For this review, take the finished solid that the model builds, in its own axes (mm). Face numbers are marked on the shaded views. A direction names the side the tool comes from. Round coordinates to 2 decimals unless told otherwise and drop trailing zeros. Write each loop counter-clockwise with the first axis right and the second up, starting at its lowest first coordinate (ties: lowest second). Pieces come first, ordered by that corner, then holes. Notation, with made-up numbers: M 55.25,56.25 L 92.25,56.25 A20 ccw 92.25,91.25 Z; hole C -10,28 d1. An arc over 180 degrees is marked long. Answer in a Markdown table with one row per item.
```python
from build123d import *

# Parameters (mm, degrees)
BOSS_EXTRUDE7_DEPTH      = 12
BOSS_EXTRUDE7_DEPTH_BACK = 12
FILLET1_R                = 10
SKETCH1_R                = 3.98
BOSS_EXTRUDE3_DEPTH      = 10
SKETCH5_R                = 1.6
CUT_EXTRUDE1_DEPTH       = 165.414111317
SKETCH6_R                = 2
CUT_EXTRUDE2_DEPTH       = 3
SKETCH7_R                = 3.98
BOSS_EXTRUDE5_DEPTH      = 10
SKETCH9_R                = 1.6
CUT_EXTRUDE3_DEPTH       = 17
SKETCH10_R               = 4
CUT_EXTRUDE4_DEPTH       = 3


with BuildPart() as part:
    # Sketch11 → Boss-Extrude7 (new, two sides: drawn at the far end of the back side and taken through both)
    with BuildSketch(Plane.XY.offset(-BOSS_EXTRUDE7_DEPTH_BACK)):
        Polygon((-86.2, 142), (-86.2, 26), (-50.2, -10), (15.8, -10), (15.8, 0), (-46.057864376, 0), (-76.2, 30.142135624), (-76.2, 142), align=None)
    extrude(amount=BOSS_EXTRUDE7_DEPTH + BOSS_EXTRUDE7_DEPTH_BACK)

    # Fillet1
    fillet1_edges = [part.edges().sort_by_distance(p)[0] for p in [
        (-81.2, 142, -12),
        (15.8, -5, -12),
        (15.8, -5, 12),
        (-81.2, 142, 12),
    ]]
    fillet(fillet1_edges, radius=FILLET1_R)

    # Sketch1 → Boss-Extrude3 (add)
    with BuildSketch(Plane(origin=(-76.2, 0, 0), x_dir=(0, 0, -1), z_dir=(1, 0, 0))):
        with Locations((0, 128)):
            Circle(SKETCH1_R)
    extrude(amount=BOSS_EXTRUDE3_DEPTH)

    # Sketch5 → Cut-Extrude1 (cut, through all)
    with BuildSketch(Plane(origin=(-66.2, 0, 0), x_dir=(0, 0, -1), z_dir=(1, 0, 0))):
        with Locations((0, 128)):
            Circle(SKETCH5_R)
    extrude(amount=-CUT_EXTRUDE1_DEPTH, mode=Mode.SUBTRACT)

    # Sketch6 → Cut-Extrude2 (cut)
    with BuildSketch(Plane.ZY.offset(86.2)):
        with Locations((0, 128)):
            Circle(SKETCH6_R)
    extrude(amount=-CUT_EXTRUDE2_DEPTH, mode=Mode.SUBTRACT)

    # Sketch7 → Boss-Extrude5 (add)
    with BuildSketch(Plane(origin=(0, 0, 0), x_dir=(1, 0, 0), z_dir=(0, 1, 0))):
        with Locations(Location((-0.08822806, 0, 0), (0, 0, 270))):
            Circle(SKETCH7_R)
    extrude(amount=BOSS_EXTRUDE5_DEPTH)

    # Sketch9 → Cut-Extrude3 (cut)
    with BuildSketch(Plane(origin=(0, 10, 0), x_dir=(1, 0, 0), z_dir=(0, 1, 0))):
        with Locations(Location((-0.08822806, 0, 0), (0, 0, 270))):
            Circle(SKETCH9_R)
    extrude(amount=-CUT_EXTRUDE3_DEPTH, mode=Mode.SUBTRACT)

    # Sketch10 → Cut-Extrude4 (cut)
    with BuildSketch(Plane.XZ.offset(10)):
        with Locations(Location((-0.08822806, 0, 0), (0, 0, 270))):
            Circle(SKETCH10_R)
    extrude(amount=-CUT_EXTRUDE4_DEPTH, mode=Mode.SUBTRACT)


solid = part.part
```
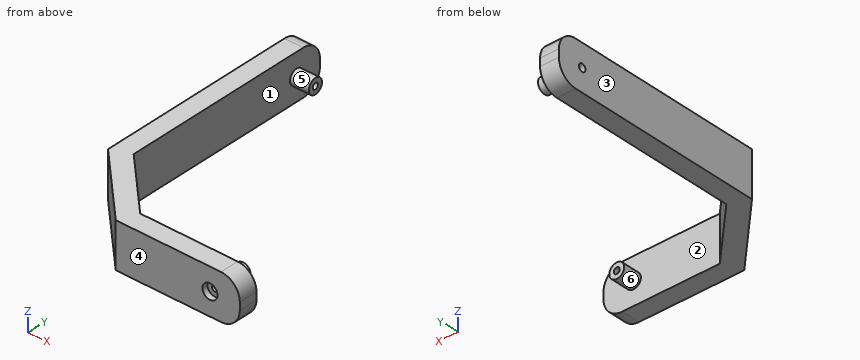
Q1. Take a section at C-C (z = 8.5). State the section outline as (x, y) points.
Found:
| item | result |
|---|---|
| outline | M -86.2,26 L -50.2,-10 L 13.4,-10 L 13.4,0 L -46.06,0 L -76.2,30.14 L -76.2,139.6 L -86.2,139.6 Z |
Q2. Take a section at A-A (y = 128). State the section outline as (x, z) points, then the cut area to 3 significant figures.
Found:
| item | result |
|---|---|
| outline | M -86.2,-12 L -76.2,-12 L -76.2,-3.98 L -66.2,-3.98 L -66.2,-1.6 L -83.2,-1.6 L -83.2,-2 L -86.2,-2 Z; M -86.2,2 L -83.2,2 L -83.2,1.6 L -66.2,1.6 L -66.2,3.98 L -76.2,3.98 L -76.2,12 L -86.2,12 Z |
| area | 253 mm² |
Q3. Take a section at B-B (z = 0). State how many separate pieces and enclosed holes the cut face has, then the cut area to 3 significant figures.
Found:
| item | result |
|---|---|
| separate pieces | 3 |
| enclosed holes | 0 |
| area | 2,260 mm² |
Q4. Mouldability with a two-part tool opening along Y and no side actions: class the marked faces 1, 2 and 3 as +Y half, -Y half, draft (parallel to the pull), parting line (faces both ways), or undercut.
Found:
| item | result |
|---|---|
| face 1 | undercut |
| face 2 | +Y half |
| face 3 | draft |
Q5. Take a section at D-D (y = 103). State the section outline as (x, z) points.
Found:
| item | result |
|---|---|
| outline | M -86.2,-12 L -76.2,-12 L -76.2,12 L -86.2,12 Z |
Q6. For probe 1 along X at (y, z) = (67.5, -10.5); probe 2 along Y at (x, z) = (-9, 2.75); probe 3 along Y at (x, z) = (1.5, -3.5), list the stretches that pass through material, from the lowest coordinate up.
Found:
| item | result |
|---|---|
| probe 1 | -86.2 to -76.2 |
| probe 2 | -10 to 0 |
| probe 3 | -7 to 10 |
Q7. Machinability: for the marked faces 4, 5 and 6, which of the approach directions +Z, -Z, +X, -X, +Y, -Y give a long, thin tool a straight path to every point of the face, cutting with its end or side? Answer none if there is none.
Found:
| item | result |
|---|---|
| face 4 | +Z, -Z, +X, -X, -Y |
| face 5 | +X |
| face 6 | +Y |
Q8. Insertion check: P1, Ø2.5, axis at x = -0.5, z = 0.5, coming from the +Y side; P2, Ø7, axis at y = 105, z = -4.5, coming from the +X side; P3, Ø1.9, axis at y = 128, z = 0, coming from the +X side; P4, Ø9, axis at y = 128, z = 0.5, coming from the +X side. Each pin has a flat end and moves straight along its axis. Give the tip position at first contact, or say it passes through.
Found:
| item | result |
|---|---|
| P1 | y = 10 |
| P2 | x = -76.2 |
| P3 | through |
| P4 | x = -66.2 |
